```python
from build123d import *

# Parameters (mm, degrees)
F0_W     = 150
F0_H     = 40
F1_DEPTH = 80
F2_W     = 65
F2_H     = 20
F3_DEPTH = 10
F4_W     = 100
F4_H     = 30
F5_DEPTH = 87.2
F6_W     = 61
F6_H     = 6
F7_DEPTH = 25


with BuildPart() as f1:
    # F0 (on Top) → F1 (new body)
    with BuildSketch(Plane.XY):
        with Locations((-0.189516, 7.814032)):
            Rectangle(F0_W, F0_H)
    extrude(amount=F1_DEPTH)

    # F2 (on face) → F3 (cut)
    with BuildSketch(Plane.XZ.offset(12.185968)):
        with Locations((1.311038, 70)):
            Rectangle(F2_W, F2_H)
    extrude(amount=-F3_DEPTH, mode=Mode.SUBTRACT)

    # F4 (on face) → F5 (cut)
    with BuildSketch(Plane.XZ.offset(12.185968)):
        with Locations((-0.189516, 32.763609)):
            Rectangle(F4_W, F4_H)
    extrude(amount=-F5_DEPTH, mode=Mode.SUBTRACT)

    # F6 (on face) → F7 (cut)
    with BuildSketch(Plane.XY.offset(60)):
        with Locations((1.311038, -7.185968)):
            Rectangle(F6_W, F6_H)
    extrude(amount=-F7_DEPTH, mode=Mode.SUBTRACT)


solid = f1.part
```
The listing builds one solid part. Answer for the finished solid, in the listing's coordinates (mm). A direction names the side the tool comes from. Round coordinates to 2 decimals unless told otherwise and drop trailing zeros. Loops run counter-clockwise (first coordinate to the right, second up) from the corner with the lowest first, then second, coordinate; pieces in that order, holes last. Notation, with made-up numbers: (9.5, 25) - (43.5, 25) arc R23 cw to (43.5, 52) - close; hole circle Ø11 at (38.5, 9.5). An arc over 180 degrees is marked (long way). Return JSON: item names as keys, results as strings. Group by question number.
1. Which of the six approach directions +Z, -Z, +X, -X, +Y, -Y give full straight-line access (tool end or side, diameter ignored) to faces 1 (the flat face through (31.811, -7, 54)), 2 (the flat face through (-1, 27.814, 48)), 3 (the flat face through (-31.189, -7, 70)), 4 (the flat face through (-50.19, 8, 33))?
2. This flat-tipped pin is pushed along its axis until it touches: P1, Ø5, axis at x = -2, y = -9.5, coming from the +Z side. Where does it stop, or does it pass through?
3. The part is cut by section B-B on y = 20. Determine the outline of the cut face in (x, z).
4. The part is cut by section A-A on z = 56. Determine the outline of the cut face in (x, y), then the cut area to 3 significant figures.
5. The part is cut by section C-C on x = -15. Determine the outline of the cut face in (y, z), then the cut area to 3 significant figures.
6. The mould has two halves that part along X. Classify faces 5 (the flat face through (-29.189, -7, 54)), 6 (the flat face through (-1, -12.186, 48)), 7 (the flat face through (-75.19, 8, 39)): pulls with the +X half, pulls with the -X half, needs draft (parallel to the pull), parting line crosses it, or undercut.
7. The part is cut by section D-D on x = 40.5. Determine the outline of the cut face in (y, z).
8. Consider probe 1 along Y at (x, z) = (-24.5, 56.5); probe 2 along Z at (x, y) = (-33, -7); probe 3 along X at (y, z) = (12, 32). Determine where each line is inside the solid, lowest interval first.
Resolved:
{
 "1": {"face 1": "+Z", "face 2": "+Z, -Z, +X, -X, +Y", "face 3": "+Z, -Y", "face 4": "+Y, -Y"},
 "2": {"P1": "stops at z = 60"},
 "3": {"outline": "(-75.19, 0) - (74.81, 0) - (74.81, 80) - (-75.19, 80) - close; hole (-50.19, 17.76) - (49.81, 17.76) - (49.81, 47.76) - (-50.19, 47.76) - close"},
 "4": {"outline": "(-75.19, -12.19) - (74.81, -12.19) - (74.81, 27.81) - (-75.19, 27.81) - close; hole (-29.19, -10.19) - (31.81, -10.19) - (31.81, -4.19) - (-29.19, -4.19) - close", "area": "5,630 mm²"},
 "5": {"outline": "(-12.19, 0) - (27.81, 0) - (27.81, 17.76) - (-12.19, 17.76) - close; (-12.19, 47.76) - (-10.19, 47.76) - (-10.19, 60) - (-12.19, 60) - close; (-4.19, 47.76) - (27.81, 47.76) - (27.81, 80) - (-2.19, 80) - (-2.19, 60) - (-4.19, 60) - close", "area": "1,730 mm²"},
 "6": {"face 5": "undercut", "face 6": "needs draft", "face 7": "pulls with the -X half"},
 "7": {"outline": "(-12.19, 0) - (27.81, 0) - (27.81, 17.76) - (-12.19, 17.76) - close; (-12.19, 47.76) - (27.81, 47.76) - (27.81, 80) - (-12.19, 80) - close"},
 "8": {"probe 1": "y = -12.19 to -10.19, -4.19 to 27.81", "probe 2": "z = 0 to 17.76, 47.76 to 80", "probe 3": "x = -75.19 to -50.19, 49.81 to 74.81"}
}
